Verification items for the finished model (mm, model axes). A direction names the side the tool comes from. Give positions to 0.01 mm unless a question says otherwise; leave off trailing zeros.
(1) Sectioned sample at A-A on x = 0. Count the separate pieces of the cut face and the enclosed holes in it, plus the area to 3 significant figures.
(2) Gauge pin test, flat ends, axial feed: pin 1 (5 mm diameter, centred on x = -4.5, y = -9, fed in from +Z); pin 2 (0.5 mm diameter, centred on x = -3.5, z = -0.5, fed in from +Y). Record the tip position at first contact, or that the pin passes through.
(3) Mould release check, pull along Y, two halves, no side actions. Record for faces 6 (the face through (-7.216, 3.389, -0.507)), 7 (the face through (-0.164, -18.477, -0.493)), 8 (the face through (-1.5, -7.4, 0)), 9 (the face through (9.107, -4.112, -0.507)): pulls with the +Y half, pulls with the -Y half, needs draft (parallel to the pull), parting line crosses it, or undercut.
(4) Access from +Z, -Z, +X, -X, +Y, -Y to the whole of each face (thin tool, end or side, straight path). Record for faces 1 (the face through (-7.7, -5.1, -0.5)), 2 (the face through (2.952, -15.6, -0.5)), 3 (the face through (-9.133, -4.074, -0.507)), 4 (the face through (3.557, -22.5, -0.5)), 5 (the face through (-8.674, -3.619, -0.493)).
(5) Scan lines: L1, parallel to Y at x = 0, z = -0.1; L2, parallel to Y at x = 3, z = -0.3; L3, parallel to Y at x = -0.25, z = -0.05. Record each from-to range of solid material in increasing order.
```python
from build123d import *

# Parameters (mm, degrees)
BOSS_EXTRUDE1_START   = -1
SKETCH1_R             = 0.8
BOSS_EXTRUDE1_DEPTH   = 1
SKETCH7_R             = 0.898548633
SKETCH7_R_2           = 0.900820611
SKETCH7_R_3           = 0.402256278
CUT_EXTRUDE9_DEPTH    = 10
F_0_80_TAPPED_HOLE2_D = 1.19126
F_0_80_TAPPED_HOLE3_D = 1.19126


with BuildPart() as part:
    # Sketch1 → Boss-Extrude1 (new body)
    with BuildSketch(Plane.XY.offset(BOSS_EXTRUDE1_START)):
        with BuildLine():
            Line((-7.655924922, -1.783859884), (-9.740911438, -2.722813484))
            Line((-9.740911438, -2.722813484), (-8.506978823, -5.462813484))
            Line((-8.506978823, -5.462813484), (-6.79791054, -4.69315104))
            add(Edge.make_bspline(
                [(-2.619308836, -7.990994312), (-4.588919021, -8.061513983), (-6.291403266, -6.510208965), (-6.79791054, -4.69315104)],
                knots=[0, 0, 0, 0, 1, 1, 1, 1], degree=3))
            add(Edge.make_bspline(
                [(-2.619308836, -7.990994312), (-2.465518072, -8.186748708), (-2.460868626, -8.496086459)],
                knots=[0.760656089, 0.760656089, 0.760656089, 1, 1, 1], degree=2))
            add(Edge.make_bspline(
                [(-2.460868626, -8.496086459), (-2.65493709, -9.55970155), (-2.927067031, -10.028695592)],
                knots=[0.505400696, 0.505400696, 0.505400696, 1, 1, 1], degree=2))
            Line((-2.927067031, -10.028695592), (-2.968919318, -20.993587767))
            Line((-2.968919318, -20.993587767), (-3.569337553, -20.993587767))
            Line((-3.569337553, -20.993587767), (-3.569337553, -23.990261353))
            Line((-3.569337553, -23.990261353), (3.556946411, -23.990261353))
            Line((3.556946411, -23.990261353), (3.556946411, -21.012656051))
            Line((3.556946411, -21.012656051), (2.952210653, -21.012656051))
            Line((2.952210653, -21.012656051), (2.952210653, -10.028695592))
            add(Edge.make_bspline(
                [(2.952210653, -10.028695592), (2.953361032, -9.730287058), (2.715766736, -8.848177203), (2.885688703, -8.273229584)],
                knots=[0, 0, 0, 0, 0.672395154, 0.672395154, 0.672395154, 0.672395154], degree=3))
            add(Edge.make_bspline(
                [(6.826829986, -4.71005972), (6.530666267, -6.607497463), (4.761489994, -8.103944733), (2.885688703, -8.273229584)],
                knots=[0, 0, 0, 0, 1, 1, 1, 1], degree=3))
            Line((6.826829986, -4.71005972), (8.498351825, -5.462813484))
            Line((8.498351825, -5.462813484), (9.73228444, -2.722813484))
            Line((9.73228444, -2.722813484), (7.707819022, -1.811114978))
            Line((7.707819022, -1.811114978), (7.717081791, -1.649283667))
            add(Edge.make_bspline(
                [(6.242730234, 6.243460256), (8.328472862, 2.657233336), (7.717081791, -1.649283667)],
                knots=[0, 0, 0, 1, 1, 1], degree=2))
            add(Edge.make_bspline(
                [(2.888581262, 8.896214027), (2.985217378, 8.879515932), (3.247765026, 8.808593113), (3.630118411, 8.642577), (4.074173184, 8.36866418), (4.721906948, 8.009989726), (5.550196572, 7.346039296), (6.012892554, 6.633136043), (6.242724869, 6.243469352), (6.242730234, 6.243460256)],
                knots=[0.680120302, 0.680120302, 0.680120302, 0.680120302, 0.700211116, 0.734681827, 0.764415496, 0.805837959, 0.884920242, 0.976406366, 0.976408502, 0.976408502, 0.976408502, 0.976408502], degree=3))
            add(Edge.make_bspline(
                [(2.888581262, 8.896214027), (2.280334466, 9.102116147), (1.335962581, 8.833175098), (-0.021268554, 8.319279629), (-1.467178457, 8.865773987), (-2.595326146, 8.990746146), (-3.261769012, 8.769028641)],
                knots=[0, 0, 0, 0, 0.291998369, 0.463731226, 0.671653294, 1, 1, 1, 1], degree=3))
            add(Edge.make_bspline(
                [(-6.978349655, 4.418537245), (-6.978341175, 4.418559118), (-6.261281728, 6.267997055), (-5.356361794, 8.204922518), (-3.261769012, 8.769028641)],
                knots=[0.183710391, 0.183710391, 0.183710391, 0.183710391, 0.183719842, 0.982772692, 0.982772692, 0.982772692, 0.982772692], degree=3))
            Line((-6.978349655, 4.418537245), (-7.459962837, 2.329545769))
            add(Edge.make_bspline(
                [(-7.459962837, 2.329545769), (-7.730690273, 0.280095873), (-7.655924922, -1.783859884)],
                knots=[0, 0, 0, 1, 1, 1], degree=2))
        make_face()
        with Locations((-4.256541488, -5.597749713)):
            Circle(SKETCH1_R, mode=Mode.SUBTRACT)
        with Locations((4.170722828, -5.597749713)):
            Circle(SKETCH1_R, mode=Mode.SUBTRACT)
        with BuildLine():
            add(Edge.make_bspline(
                [(-1.804027034, -5.787976133), (0.02164308, -10.328457974), (1.839505032, -5.833009783)],
                knots=[0, 0, 0, 1, 1, 1], degree=2))
            Line((-1.804027034, -5.787976133), (-1.962380096, -5.114496208))
            add(Edge.make_bspline(
                [(-1.962380096, -5.114496208), (-2.941705535, -4.714827932), (-4.153358989, -4.614522903), (-4.895639487, -3.761606791)],
                knots=[0, 0, 0, 0, 1, 1, 1, 1], degree=3))
            add(Edge.make_bspline(
                [(-4.256541488, 6.424442026), (-5.024773734, 5.435848631), (-5.987106297, 2.960839001), (-5.849347194, -0.56805471), (-5.37593872, -2.947032062), (-4.895639487, -3.761606791)],
                knots=[0, 0, 0, 0, 0.272445914, 0.556070127, 0.771313395, 0.771313395, 0.771313395, 0.771313395], degree=3))
            add(Edge.make_bspline(
                [(-3.261769012, 7.15739827), (-3.8717566, 6.941904365), (-4.256541488, 6.424442026)],
                knots=[0, 0, 0, 1, 1, 1], degree=2))
            add(Edge.make_bspline(
                [(-3.261769012, 7.15739827), (-3.163039034, 7.19003027), (-2.117380019, 7.410646221), (0.07712388, 4.390116457), (2.247368009, 7.809908036), (3.370301543, 6.988790875), (3.593464255, 6.757042923)],
                knots=[0.223669574, 0.223669574, 0.223669574, 0.223669574, 0.250320471, 0.504380952, 0.76319614, 0.835276292, 0.835276292, 0.835276292, 0.835276292], degree=3))
            add(Edge.make_bspline(
                [(3.593464255, 6.757042923), (5.644175861, 5.268051013), (6.650840286, 1.422043117), (5.831780767, -2.644018853), (5.005569013, -3.761606791)],
                knots=[0, 0, 0, 0, 0.480405077, 0.775338814, 0.775338814, 0.775338814, 0.775338814], degree=3))
            add(Edge.make_bspline(
                [(1.979863992, -5.114496208), (3.102537491, -5.017783712), (4.162687131, -4.499401159), (5.005569013, -3.761606791)],
                knots=[0, 0, 0, 0, 1, 1, 1, 1], degree=3))
            Line((1.979863992, -5.114496208), (1.839505032, -5.833009783))
        make_face(mode=Mode.SUBTRACT)
        with Locations((0.012809238, 7.182899015)):
            Circle(SKETCH1_R, mode=Mode.SUBTRACT)
    extrude(amount=BOSS_EXTRUDE1_DEPTH)

    # Sketch7 → Cut-Extrude9 (cut)
    with BuildSketch(Plane.XY):
        with Locations((-0.047392103, -19.368039034)):
            Circle(SKETCH7_R)
        with Locations((-0.046989341, -16.376260671)):
            Circle(SKETCH7_R_2)
        with Locations((-1.287320407, -11.446362098)):
            Circle(SKETCH7_R_3)
    extrude(amount=-CUT_EXTRUDE9_DEPTH, mode=Mode.SUBTRACT)

    # #0-80 Tapped Hole2 (through all)
    with Locations(Plane(origin=(0, 0, -1), x_dir=(-1, 0, 0), z_dir=(0, 0, -1))):
        with Locations((-7.922698165, -3.556993775)):
            Hole(F_0_80_TAPPED_HOLE2_D / 2)

    # #0-80 Tapped Hole3 (through all)
    with Locations(Plane(origin=(0, 0, -1), x_dir=(-1, 0, 0), z_dir=(0, 0, -1))):
        with Locations((8.078988794, -3.645070301)):
            Hole(F_0_80_TAPPED_HOLE3_D / 2)


solid = part.part
```
Ans:
1. separate pieces: 5
1. enclosed holes: 0
1. area: 13.3 mm2
2. pin 1: stops at z = 0
2. pin 2: stops at y = 8.77
3. face 6: pulls with the +Y half
3. face 7: undercut
3. face 8: needs draft
3. face 9: pulls with the -Y half
4. face 1: +Z, -Z, -Y
4. face 2: +Z, -Z, +X
4. face 3: +Z, -Z, -X, -Y
4. face 4: +Z, -Z, +X, -Y
4. face 5: +Z, -Z
5. L1: y = -23.99 to -20.27, -18.47 to -17.28, -15.48 to -8.07, 5.86 to 6.38, 7.98 to 8.47
5. L2: y = -23.99 to -21.01, -8.26 to -4.91, 7.18 to 8.87
5. L3: y = -23.99 to -20.24, -18.49 to -17.25, -15.5 to -8.02, 5.88 to 6.43, 7.94 to 8.48
